from build123d import *

# Parameters (mm, degrees)
F0_R     = 5.5
F1_DEPTH = 2
F2_R     = 2.8
F3_DEPTH = 5
F2_R_2   = 5.15
F2_R_3   = 4.15
F4_DEPTH = 7
F5_SIZE2 = 1
F5_SIZE  = 1
F6_R     = 0.99999
F7_SIZE  = 1


# Not quite as in the source:
# - a fillet or chamfer is up to 0.001 mm smaller than in the source, because OpenCascade refuses the exact size


with BuildPart() as f1:
    # F0 (on Top) → F1 (new body)
    with BuildSketch(Plane.XY):
        Circle(F0_R)
    extrude(amount=F1_DEPTH)

    # F2 (on face) → F3 (join)
    with BuildSketch(Plane.XY.offset(2)):
        Circle(F2_R)
    extrude(amount=F3_DEPTH)

    # F2 (on face) → F4 (join)
    with BuildSketch(Plane.XY.offset(2)):
        Circle(F2_R_2)
        Circle(F2_R_3, mode=Mode.SUBTRACT)
    extrude(amount=F4_DEPTH)

    # F5
    f5_edges = [f1.edges().sort_by_distance(p)[0] for p in [
        (-2.8, 0, 7),
    ]]
    chamfer(f5_edges, length=F5_SIZE, length2=F5_SIZE2)

    # F6 (radius 1 in the source; OpenCascade refuses exactly that, so slightly less here)
    f6_edges = [f1.edges().sort_by_distance(p)[0] for p in [
        (-5.15, 0, 9),
    ]]
    fillet(f6_edges, radius=F6_R)

    # F7
    f7_edges = [f1.edges().sort_by_distance(p)[0] for p in [
        (-5.5, 0, 0),
    ]]
    chamfer(f7_edges, length=F7_SIZE)


solid = f1.part
Geometry: final body of the model. Coordinates: model frame, mm. A direction names the side the tool comes from. Give positions to 0.01 mm unless a question says otherwise; leave off trailing zeros. Write each loop counter-clockwise with the first axis right and the second up, starting at its lowest first coordinate (ties: lowest second). Pieces come first, ordered by that corner, then holes. Notation, with made-up numbers: (55, 88) -> (101, 88) arc R16 cw to (101, 96) -> close; hole circle Ø4 at (10.5, 14). An arc over 180 degrees is marked (long way). Answer as a JSON object with one key per item and string values.
1. Cut plane A-A on z = 2.25. Output: boundary loops of the cut face in (x, y).
Ans:
{"outline": "circle Ø10.3 at (0, 0); circle Ø5.6 at (0, 0); hole circle Ø8.3 at (0, 0)"}
2. Access query for faces 4 (the cylindrical face through (-1.19, -5.37, 1.49)), 5 (the flat face through (3, -1, 2)). Directions: +Z, -Z, +X, -X, +Y, -Y. A direction counts if a zero-diameter tool reaches every point of the face in a straight line with its end or side. Return the directions, or none.
Ans:
{"face 4": "+Z, -Z", "face 5": "+Z"}
3. Mould query, pull axis X, two halves, no side actions, for faces 1 (the flat face through (0, 0, 7)), 2 (the flat face through (0, 0, 0)), 3 (the cylindrical face through (4.91, 1.55, 4.96)). Classes: pulls with the +X half, pulls with the -X half, needs draft (parallel to the pull), parting line crosses it, or undercut.
Ans:
{"face 1": "undercut", "face 2": "needs draft", "face 3": "parting line crosses it"}
4. Ray query, probe 1 along Y at (x, z) = (0, 5.5); probe 2 along Y at (x, z) = (0, 6.25); probe 3 along X at (y, z) = (-2.5, 5.75). Return the intervals inside material, ascending. Write a range as from..to.
Ans:
{"probe 1": "y = -5.15..-4.15, -2.8..2.8, 4.15..5.15", "probe 2": "y = -5.15..-4.15, -2.55..2.55, 4.15..5.15", "probe 3": "x = -4.5..-3.31, -1.26..1.26, 3.31..4.5"}
5. Contact query for flat-ended pins moving along their axis: pin 1 (2 mm diameter, centred on x = 3.5, z = 2, fed in from +Y); pin 2 (3.5 mm diameter, centred on x = 0, y = -1.5, fed in from +Z); pin 3 (5 mm diameter, centred on x = -1, z = 7.5, fed in from -Y). Output: stop coordinate, or through.
Ans:
{"pin 1": "stops at y = 4.9", "pin 2": "stops at z = 7", "pin 3": "stops at y = -5.15"}
6. Cut plane D-D on z = 7.75. Output: boundary loops of the cut face in (x, y).
Ans:
{"outline": "circle Ø10.3 at (0, 0); hole circle Ø8.3 at (0, 0)"}
